```python
from build123d import *

# Parameters (mm, degrees)
CROQUIS1_R              = 3.556
SALIENTE_EXTRUIR1_DEPTH = 3.1242
SALIENTE_EXTRUIR3_START = -3.1242
SALIENTE_EXTRUIR3_DEPTH = 3.1242
CROQUIS3_R              = 1.016
CORTAR_EXTRUIR1_DEPTH   = 45.81344142


with BuildPart() as part:
    # Croquis1 → Saliente-Extruir1 (new body)
    with BuildSketch(Plane.XY):
        with BuildLine():
            Line((9.525, 0), (9.525, 33.3375))
            ThreePointArc((9.525, 33.3375), (0, 42.8625), (-9.525, 33.3375))
            Line((-9.525, 33.3375), (-9.525, 0))
            ThreePointArc((-9.525, 0), (0, -9.525), (9.525, 0))
        make_face()
        Circle(CROQUIS1_R, mode=Mode.SUBTRACT)
        with BuildLine():
            ThreePointArc((-6.35, 26.9875), (0, 20.6375), (6.35, 26.9875))
            Line((6.35, 26.9875), (6.35, 33.3375))
            ThreePointArc((6.35, 33.3375), (0, 39.6875), (-6.35, 33.3375))
            Line((-6.35, 33.3375), (-6.35, 26.9875))
        make_face(mode=Mode.SUBTRACT)
        with BuildLine():
            ThreePointArc((1.524, 12.7), (0, 14.224), (-1.524, 12.7))
            Line((-1.524, 12.7), (-1.524, 6.35))
            ThreePointArc((-1.524, 6.35), (0, 4.826), (1.524, 6.35))
            Line((1.524, 6.35), (1.524, 12.7))
        make_face(mode=Mode.SUBTRACT)
    extrude(amount=SALIENTE_EXTRUIR1_DEPTH)

    # Croquis2 → Saliente-Extruir3 (add)
    with BuildSketch(Plane.XY.offset(3.1242).offset(SALIENTE_EXTRUIR3_START)):
        with BuildLine():
            ThreePointArc((-9.525, 33.3375), (-6.735192091, 40.072692091), (0, 42.8625))
            ThreePointArc((0, 42.8625), (-8.980256121, 39.142756121), (-12.7, 30.1625))
            ThreePointArc((-12.7, 30.1625), (-12.294493201, 27.412869343), (-11.1125, 24.897358145))
            ThreePointArc((-11.1125, 24.897358145), (-9.930506799, 22.381846948), (-9.525, 19.632216291))
            Line((-9.525, 19.632216291), (-9.525, 29.1465))
            ThreePointArc((-9.525, 29.1465), (-10.541, 30.1625), (-9.525, 31.1785))
            Line((-9.525, 31.1785), (-9.525, 33.3375))
        make_face()
        with BuildLine():
            ThreePointArc((12.7, 30.1625), (8.980256121, 39.142756121), (0, 42.8625))
            ThreePointArc((0, 42.8625), (6.735192091, 40.072692091), (9.525, 33.3375))
            Line((9.525, 33.3375), (9.525, 31.1785))
            ThreePointArc((9.525, 31.1785), (10.541, 30.1625), (9.525, 29.1465))
            Line((9.525, 29.1465), (9.525, 19.632216291))
            ThreePointArc((9.525, 19.632216291), (9.930506799, 22.381846948), (11.1125, 24.897358145))
            ThreePointArc((11.1125, 24.897358145), (12.294493201, 27.412869343), (12.7, 30.1625))
        make_face()
    extrude(amount=SALIENTE_EXTRUIR3_DEPTH)

    # Croquis3 → Cortar-Extruir1 (cut, through all)
    with BuildSketch(Plane.XY.offset(3.1242)):
        with Locations((-9.525, 30.1625)):
            Circle(CROQUIS3_R)
        with Locations((9.525, 30.1625)):
            Circle(CROQUIS3_R)
    extrude(amount=-CORTAR_EXTRUIR1_DEPTH, mode=Mode.SUBTRACT)


solid = part.part
```
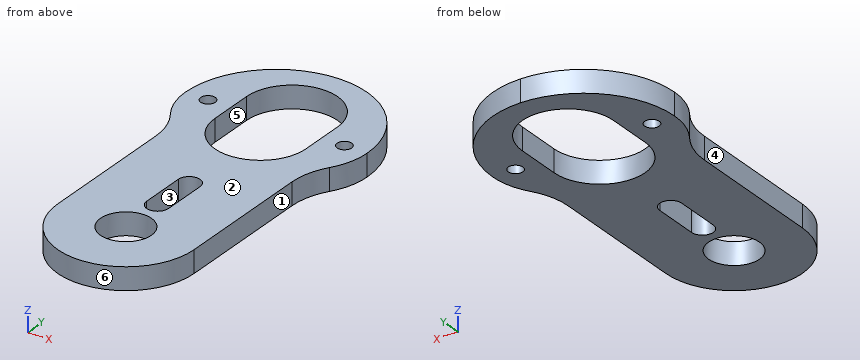
For this review, take the finished solid that the model builds, in its own axes (mm). Face numbers are marked on the shaded views. A direction names the side the tool comes from. Coordinates: 2 decimals unless noted, no trailing zeros. Write each loop counter-clockwise with the first axis right and the second up, starting at its lowest first coordinate (ties: lowest second). Pieces come first, ordered by that corner, then holes. Notation, with made-up numbers: (37.5, 29) - (88.5, 29) arc R18 ccw to (88.5, 51) - close; hole circle Ø6 at (83.5, 71.5). An arc over 180 degrees is marked (long way). Put each result on its own line as item: value.
1. Wall thickness on probe 1 along Y at (x, z) = (-1.75, 1.35); probe 2 along X at (y, z) = (9, 1.3) (3 decimals); probe 3 along Y at (x, z) = (-2, 1.65): over which ranges is each line inside the solid? List them lowest first.
Values found:
probe 1: -9.36 to -3.1, 3.1 to 20.88, 39.44 to 42.74
probe 2: -9.525 to -1.524, 1.524 to 9.525
probe 3: -9.31 to -2.94, 2.94 to 20.96, 39.36 to 42.7
2. Mouldability with a two-part tool opening along X and no side actions: class the marked faces 1, 2 and 3 as released by +X, released by -X, zero draft, split by the parting line, or undercut.
Values found:
face 1: released by +X
face 2: zero draft
face 3: undercut
3. Machinability: for the marked faces 4, 5 and 6, which of the approach directions +Z, -Z, +X, -X, +Y, -Y give a long, thin tool a straight path to every point of the face, cutting with its end or side? Answer none if there is none.
Values found:
face 4: +Z, -Z, -X, -Y
face 5: +Z, -Z
face 6: +Z, -Z, -Y
4. Add section B-B, the plane z = 1.85. Count the separate pieces of the cut face and the enclosed holes in it, then the cut area to 3 significant figures.
Values found:
separate pieces: 1
enclosed holes: 5
area: 724 mm²
5. Add section C-C, the plane x = 0.5. Give the boundary of the cut face in (y, z).
Values found:
outline: (-9.51, 0) - (-3.52, 0) - (-3.52, 3.12) - (-9.51, 3.12) - close; (3.52, 0) - (4.91, 0) - (4.91, 3.12) - (3.52, 3.12) - close; (14.14, 0) - (20.66, 0) - (20.66, 3.12) - (14.14, 3.12) - close; (39.67, 0) - (42.85, 0) - (42.85, 3.12) - (39.67, 3.12) - close
6. Add section D-D, the plane x = -4.5. Give the boundary of the cut face in (y, z).
Values found:
outline: (-8.39, 0) - (22.51, 0) - (22.51, 3.12) - (-8.39, 3.12) - close; (37.82, 0) - (42.04, 0) - (42.04, 3.12) - (37.82, 3.12) - close
7. For pin 1 (5.5 mm diameter, centred on x = 0, y = 0, fed in from +Z) (1 decimal); pin 2 (1.6 mm diameter, centred on y = 9.5, z = 2, fed in from -X) (3 decimals); pin 3 (0.9 mm diameter, centred on y = 5, z = 2, fed in from +X) (3 decimals); pin 4 (0.9 mm diameter, centred on y = 31.5, z = 1.5, fed in from -X), all flat-tipped, find the tip position at first contact; note any pin that passes through.
Values found:
pin 1: through
pin 2: x = -9.525
pin 3: x = 9.525
pin 4: x = -12.67
8. Add section A-A, the plane y = 7. Give the boundary of the cut face in (x, z) (3 decimals), then the cut area to 3 significant figures.
Values found:
outline: (-9.525, 0) - (-1.524, 0) - (-1.524, 3.124) - (-9.525, 3.124) - close; (1.524, 0) - (9.525, 0) - (9.525, 3.124) - (1.524, 3.124) - close
area: 50.0 mm²
